The model under review builds one solid part; all positions refer to its coordinate system, in mm. Face numbers are marked on the shaded views. A direction names the side the tool comes from. Coordinates: 2 decimals unless noted, no trailing zeros. Write each loop counter-clockwise with the first axis right and the second up, starting at its lowest first coordinate (ties: lowest second). Pieces come first, ordered by that corner, then holes. Notation, with made-up numbers: (31.25, -37.5) - (86.25, -37.5) arc R36 ccw to (86.25, -1.5) - close; hole circle Ø5 at (13.5, 64). An arc over 180 degrees is marked (long way). Put each result on its own line as item: value.
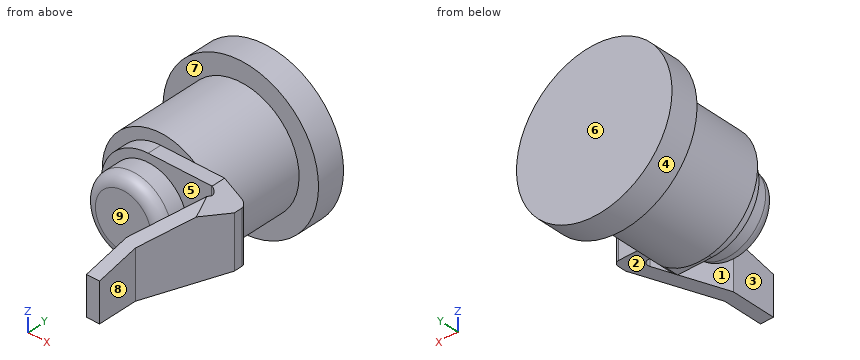
from build123d import *

# Parameters (mm, degrees)
SKETCH1_R           = 14
BOSS_EXTRUDE1_DEPTH = 5
SKETCH2_R           = 10.5
BOSS_EXTRUDE2_DEPTH = 16
SKETCH3_R           = 8.5
BOSS_EXTRUDE3_DEPTH = 2.5
SKETCH4_R           = 7
BOSS_EXTRUDE4_DEPTH = 5
FILLET1_R           = 2
BOSS_EXTRUDE5_START = -2.5
BOSS_EXTRUDE5_DEPTH = 2.5
BOSS_EXTRUDE7_DEPTH = 17
FILLET3_R           = 1
CUT_EXTRUDE1_REACH  = 53.435
CUT_EXTRUDE2_DEPTH  = 20
SKETCH10_W          = 8.800813703
SKETCH10_H          = 15.870840907
CUT_EXTRUDE3_DEPTH  = 10


with BuildPart() as part:
    # Sketch1 → Boss-Extrude1 (new body)
    with BuildSketch(Plane(origin=(0, 0, 0), x_dir=(1, 0, 0), z_dir=(0, 1, 0))):
        with Locations(Location((0, 0, 0), (0, 0, 270))):
            Circle(SKETCH1_R)
    extrude(amount=BOSS_EXTRUDE1_DEPTH)

    # Sketch2 → Boss-Extrude2 (add)
    with BuildSketch(Plane.XZ):
        with Locations(Location((0, 0, 0), (0, 0, 270))):
            Circle(SKETCH2_R)
    extrude(amount=BOSS_EXTRUDE2_DEPTH)

    # Sketch3 → Boss-Extrude3 (add)
    with BuildSketch(Plane.XZ.offset(16)):
        with Locations(Location((0, 0, 0), (0, 0, 270))):
            Circle(SKETCH3_R)
    extrude(amount=BOSS_EXTRUDE3_DEPTH)

    # Sketch4 → Boss-Extrude4 (add)
    with BuildSketch(Plane.XZ.offset(18.5)):
        with Locations(Location((0, 0, 0), (0, 0, 270))):
            Circle(SKETCH4_R)
    extrude(amount=BOSS_EXTRUDE4_DEPTH)

    # Fillet1
    fillet1_edges = [part.edges().sort_by_distance(p)[0] for p in [
        (0, -23.5, 7),
    ]]
    fillet(fillet1_edges, radius=FILLET1_R)

    # Sketch5 → Boss-Extrude5 (add)
    with BuildSketch(Plane.XZ.offset(18.5).offset(BOSS_EXTRUDE5_START)):
        with BuildLine():
            Line((15.5, 8.5), (0, 8.5))
            ThreePointArc((0, 8.5), (6.01040764, 6.01040764), (8.5, 0))
            ThreePointArc((8.5, 0), (6.01040764, -6.01040764), (0, -8.5))
            Line((0, -8.5), (15.5, -8.5))
            Line((15.5, -8.5), (15.5, 8.5))
        make_face()
    extrude(amount=BOSS_EXTRUDE5_DEPTH)

    # Sketch7 → Boss-Extrude7 (add)
    with BuildSketch(Plane.XY.offset(8.5)):
        Polygon((15.5, -18.5), (10.36969785, -32.595389312), (10.36969785, -39.740338953), (8.020466298, -39.740338953), (8.020466298, -31.740338953), (12.839555569, -18.5), align=None)
    extrude(amount=-BOSS_EXTRUDE7_DEPTH)

    # Fillet3
    fillet3_edges = [part.edges().sort_by_distance(p)[0] for p in [
        (15.5, -16, 0),
        (12.839555569, -18.5, 0),
    ]]
    fillet(fillet3_edges, radius=FILLET3_R)

    # Cut-Extrude1: up to this face of the body (flat: up to its plane)
    cut_extrude1_end = Plane(part.part.faces().sort_by_distance((8.020466298, -35.740338953, 0))[0])
    # Sketch8 → Cut-Extrude1 (cut, up to the picked face)
    with BuildSketch(Plane(origin=(15.5, 0, 0), x_dir=(0, 0, -1), z_dir=(1, 0, 0)), mode=Mode.PRIVATE) as cut_extrude1_sk1:
        Polygon((-3.5, -39.740338953), (-8.5, -18.5), (-8.5, -32.595389312), (-8.5, -39.740338953), align=None)
    cut_extrude1_tool1 = split(extrude(cut_extrude1_sk1.sketch, amount=-CUT_EXTRUDE1_REACH, mode=Mode.PRIVATE), bisect_by=cut_extrude1_end, keep=Keep.BOTH, mode=Mode.PRIVATE)
    # Sketch8 → Cut-Extrude1 (cut, up to the picked face)
    with BuildSketch(Plane(origin=(15.5, 0, 0), x_dir=(0, 0, -1), z_dir=(1, 0, 0)), mode=Mode.PRIVATE) as cut_extrude1_sk2:
        Polygon((8.5, -32.595389312), (8.5, -18.5), (3.5, -39.740338953), (8.5, -39.740338953), align=None)
    cut_extrude1_tool2 = split(extrude(cut_extrude1_sk2.sketch, amount=-CUT_EXTRUDE1_REACH, mode=Mode.PRIVATE), bisect_by=cut_extrude1_end, keep=Keep.BOTH, mode=Mode.PRIVATE)
    add(cut_extrude1_tool1.solids().sort_by(Axis((15.5, -32.660226, 6.833333), (-1, 0, 0)))[0], mode=Mode.SUBTRACT)
    add(cut_extrude1_tool2.solids().sort_by(Axis((15.5, -32.660226, -6.833333), (-1, 0, 0)))[0], mode=Mode.SUBTRACT)

    # Sketch9 → Cut-Extrude2 (cut)
    with BuildSketch(Plane(origin=(0, -16, 0), x_dir=(1, 0, 0), z_dir=(0, 1, 0))):
        Polygon((14.5, 8.5), (14.5, 6.625), (15.5, 6), (15.5, 8.5), align=None)
        Polygon((14.5, 8.5), (11.5, 8.5), (14.5, 6.625), align=None)
        Polygon((14.5, -6.625), (14.5, -8.5), (15.5, -8.5), (15.5, -6), align=None)
        Polygon((14.5, -6.625), (11.5, -8.5), (14.5, -8.5), align=None)
        Polygon((14.5, 6.625), (14.5, 3.5), (15.5, 3.5), (15.5, 6), align=None)
        Polygon((11.5, 8.5), (11.5, 3.5), (14.5, 3.5), (14.5, 6.625), align=None)
        with BuildLine():
            ThreePointArc((6.164414003, 8.5), (8.412032608, 6.283924522), (9.899494937, 3.5))
            Line((9.899494937, 3.5), (10.36969785, 3.5))
            Line((10.36969785, 3.5), (11.5, 3.5))
            Line((11.5, 3.5), (11.5, 8.5))
            Line((11.5, 8.5), (6.164414003, 8.5))
        make_face()
    extrude(amount=-CUT_EXTRUDE2_DEPTH, mode=Mode.SUBTRACT)

    # Sketch10 → Cut-Extrude3 (cut)
    with BuildSketch(Plane(origin=(10.36969785, 0, 0), x_dir=(0, 0, -1), z_dir=(1, 0, 0))):
        with Locations((7.900406852, -31.8049185)):
            Rectangle(SKETCH10_W, SKETCH10_H)
    extrude(amount=-CUT_EXTRUDE3_DEPTH, mode=Mode.SUBTRACT)


solid = part.part
1. Consider section D-D on z = -10. State the section outline as (x, y) points.
Determined:
outline: (-9.8, 0) - (-3.2, 0) - (-3.2, -16) - (3.2, -16) - (3.2, 0) - (9.8, 0) - (9.8, 5) - (-9.8, 5) - close
2. For pin 1 Ø2 at (x, y) = (12.5, -27.5) entering from -Z; pin 2 Ø2 at (y, z) = (-4.5, -0.5) entering from -X; pin 3 Ø13.5 at (x, z) = (-1.5, -4) entering from -Y, all flat-tipped, find the tip position at first contact; note any pin that passes through.
Determined:
pin 1: stops at z = -3.5
pin 2: stops at x = -10.5
pin 3: stops at y = -23.5
3. To check wall thickness, follow probe 1 along Y at (x, z) = (1.75, 0.75); probe 2 along Y at (x, z) = (-1.5, -7.75); probe 3 along X at (y, z) = (-36, 2.5). State the ranges of each line that lie inside material, in increasing order.
Determined:
probe 1: y = -23.5 to 5
probe 2: y = -18.5 to 5
probe 3: x = 8.02 to 10.37
4. The part is to be moulded in two halves that separate along Y. For the marked faces 6, 7, 8 and 9, say which applies: +Y half, -Y half, draft (parallel to the pull), parting line (faces both ways), or undercut.
Determined:
face 6: +Y half
face 7: undercut
face 8: draft
face 9: -Y half
5. Consider section A-A on z = 0. State the section outline as (x, y) points, plus the area to 3 significant figures.
Determined:
outline: (-14, 0) - (-10.5, 0) - (-10.5, -16) - (-8.5, -16) - (-8.5, -18.5) - (-7, -18.5) - (-7, -21.5) arc R2 ccw to (-5, -23.5) - (5, -23.5) arc R2 ccw to (7, -21.5) - (7, -18.5) - (11.41, -18.5) arc R1 cw to (12.35, -19.84) - (8.02, -31.74) - (8.02, -39.74) - (10.37, -39.74) - (10.37, -32.6) - (15.5, -18.5) - (15.5, -17) arc R1 ccw to (14.5, -16) - (10.5, -16) - (10.5, 0) - (14, 0) - (14, 5) - (-14, 5) - close
area: 659 mm^2
6. Machinability: for the marked faces 1, 2, 3, 4 and 5, which of the approach directions +Z, -Z, +X, -X, +Y, -Y give a long, thin tool a straight path to every point of the face, cutting with its end or side? Answer none if there is none.
Determined:
face 1: +Z, -Z
face 2: -Z, +X, -Y
face 3: +Z, -Z, -X, -Y
face 4: +Y
face 5: none
7. Consider section C-C on y = -5.5. State the section outline as (x, z) points, plus the area to 3 significant figures.
Determined:
outline: circle Ø21 at (0, 0)
area: 346 mm^2
8. Consider section B-B on x = -8. State the section outline as (y, z) points.
Determined:
outline: (-18.5, -2.87) - (-16, -2.87) - (-16, -6.8) - (0, -6.8) - (0, -11.49) - (5, -11.49) - (5, 11.49) - (0, 11.49) - (0, 6.8) - (-16, 6.8) - (-16, 2.87) - (-18.5, 2.87) - close
